```python
from build123d import *

# Parameters (mm, degrees)
BOSS_EXTRUDE1_DEPTH = 10
SKETCH5_W           = 19.453021512
SKETCH5_H           = 38.694970839
BOSS_EXTRUDE2_DEPTH = 85.63051792
SKETCH6_R           = 22
SKETCH6_R_2         = 19.780571117
BOSS_EXTRUDE5_DEPTH = 7.660427645
FILLET10_R          = 2.5
FILLET11_R          = 2.5


with BuildPart() as part:
    # Sketch1 → Boss-Extrude1 (new body)
    with BuildSketch(Plane(origin=(0, 0, 0), x_dir=(1, 0, 0), z_dir=(0, 1, 0))):
        with BuildLine():
            Line((0, 24.518151768), (0, 38.694970839))
            Line((0, 38.694970839), (147.451699193, 38.694970839))
            Line((147.451699193, 38.694970839), (147.451699193, 0))
            Line((147.451699193, 0), (0, 0))
            Line((0, 0), (0, 15.74024552))
            add(Edge.make_bspline(
                [(0, 15.74024552), (2.540846011, 20.138217128), (14.801575787, 5.452312854), (15.995670115, 19.711234682)],
                knots=[0, 0, 0, 0, 1, 1, 1, 1], degree=3))
            add(Edge.make_bspline(
                [(0, 24.518151768), (3.025411482, 20.257839716), (15.777331359, 32.77346932), (15.995670115, 19.711234682)],
                knots=[0, 0, 0, 0, 1, 1, 1, 1], degree=3))
        make_face()
    extrude(amount=BOSS_EXTRUDE1_DEPTH)

    # Sketch5 → Boss-Extrude2 (add)
    with BuildSketch(Plane.XZ):
        with Locations((137.725188437, -19.347485419)):
            Rectangle(SKETCH5_W, SKETCH5_H)
    extrude(amount=BOSS_EXTRUDE2_DEPTH)

    # Sketch6 → Boss-Extrude5 (add)
    with BuildSketch(Plane.ZY.offset(-127.998677681)):
        with Locations(Location((-19.34748542, -65.278, 0), (0, 0, 151.573820003))):
            Circle(SKETCH6_R)
        with Locations(Location((-19.34748542, -65.278, 0), (0, 0, 192.011596254))):
            Circle(SKETCH6_R_2, mode=Mode.SUBTRACT)
    extrude(amount=BOSS_EXTRUDE5_DEPTH)

    # Fillet10
    # the kernel refuses this fillet: 2.5 mm, written as the material it takes off along each edge
    with BuildSketch(Plane(origin=(127.998677681, -65.278, -19.34748542), x_dir=(0, 0.7021921970481064, -0.711987442589231), z_dir=(0, 0.711987442589231, 0.7021921970481064))) as fillet10_piece_1_section:
        with BuildLine():
            CenterArc((19.5, 2.48420608), FILLET10_R, 276.443791757, 83.556208243)
            Line((22, 2.48420608), (22, 0))
            Line((22, 0), (19.780571117, 0))
        make_face()
    fillet10_piece_1 = revolve(axis=Axis((127.998677681, -65.278, -19.34748542), (-1, 0, 0)), revolution_arc=89.20629991, mode=Mode.PRIVATE)
    fillet10_piece_1 = split(fillet10_piece_1, bisect_by=Plane(origin=(127.183421673, -65.278, -38.694970839), z_dir=(0, 0, -1)), keep=Keep.TOP, mode=Mode.PRIVATE)
    add(fillet10_piece_1, mode=Mode.SUBTRACT)

    # Fillet11
    # the kernel refuses this fillet: 2.5 mm, written as the material it takes off along each edge
    with BuildSketch(Plane(origin=(127.998677681, -65.278, -19.34748542), x_dir=(0, -0.7815945319539552, -0.6237868126368795), z_dir=(0, 0.6237868126368795, -0.7815945319539552))) as fillet11_piece_1_section:
        with BuildLine():
            CenterArc((22 - FILLET11_R, FILLET11_R), FILLET11_R, 270, 90)
            Line((22, FILLET11_R), (22, 0))
            Line((22, 0), (22 - FILLET11_R, 0))
        make_face()
    fillet11_piece_1 = revolve(axis=Axis((127.998677681, -65.278, -19.34748542), (-1, 0, 0)), revolution_arc=77.186396047, mode=Mode.PRIVATE)
    fillet11_piece_1 = split(fillet11_piece_1, bisect_by=Plane(origin=(127.364659544, -85.63051792, -19.347486624), z_dir=(0, -1, 0)), keep=Keep.TOP, mode=Mode.PRIVATE)
    add(fillet11_piece_1, mode=Mode.SUBTRACT)


solid = part.part
```
Build history of the part. All positions in model axes, mm. A direction names the side the tool comes from. Give positions to 0.01 mm unless a question says otherwise; leave off trailing zeros. Loops run counter-clockwise (first coordinate to the right, second up) from the corner with the lowest first, then second, coordinate; pieces in that order, holes last. Notation, with made-up numbers: (77.25, 0) -> (127.25, 0) arc R17 ccw to (127.25, 11) -> close; hole circle Ø2 at (-21, 46). An arc over 180 degrees is marked (long way). One line per question, with ' | ' between items.
Q1. Cut at C-C, the plane y = -65. Count the separate pieces of the cut face and the enclosed holes in it, plus the area to 3 significant figures.
Filled sheet:
separate pieces: 3 | enclosed holes: 0 | area: 785 mm²
Q2. Tool access for faces 1 (the flat face through (127.999, -83, -3)), 2 (the flat face through (120.338, -81, -7)), 3 (the flat face through (127.999, -83, -36)): list every direction of +Z, -Z, +X, -X, +Y, -Y with a clear straight run to the whole face (end or side of a thin tool).
Filled sheet:
face 1: +Z, -X, -Y | face 2: +Z, -Z, -X, -Y | face 3: -Z, -X, -Y
Q3. Cut at A-A, the plane y = -77.5. Write the cut outline in (x, z), plus the area to 3 significant figures.
Filled sheet:
outline: (120.34, -37.64) -> (128, -37.64) -> (128, -38.69) -> (147.45, -38.69) -> (147.45, 0) -> (128, 0) -> (128, -1.05) -> (120.34, -1.05) -> (120.34, -3.79) -> (128, -3.79) -> (128, -34.9) -> (120.34, -34.9) -> close | area: 795 mm²
Q4. Pull direction Z, two halves, no side cores. Call faces 4 (the flat face through (127.999, -65, -20)), 5 (the flat face through (129, -23, -38.695)), 6 (the flat face through (127.999, -21, -20)): pulls with the +Z half, pulls with the -Z half, needs draft (parallel to the pull), parting line crosses it, or undercut.
Filled sheet:
face 4: undercut | face 5: pulls with the -Z half | face 6: needs draft
Q5. Cut at D-D, the plane x = 36. Write the cut outline in (y, z).
Filled sheet:
outline: (0, -38.69) -> (10, -38.69) -> (10, 0) -> (0, 0) -> close
Q6. Drill centre lines: line 1 along Y through (x, z) = (123, -18); line 2 along Y through (x, z) = (125, -8.5); line 3 along Y through (x, z) = (131.5, -15). Where is each one in solid material? Low to high. Write a range as [from, to].
Filled sheet:
line 1: y = [-87.24, -85.01], [-45.54, -43.32], [0, 10] | line 2: y = [-84.42, -81.82], [-48.74, -46.14], [0, 10] | line 3: y = [-85.63, 10]
Q7. Drop flat-ended pins along their axis: pin 1 (12 mm diameter, centred on x = 65, z = -32, fed in from -Y); pin 2 (8 mm diameter, centred on y = -81, z = -32.5, fed in from -X); pin 3 (1.3 mm diameter, centred on y = -70, z = 1.5, fed in from +X). Give the stop position or say it passes through.
Filled sheet:
pin 1: stops at y = 0 | pin 2: stops at x = 120.34 | pin 3: stops at x = 128
Q8. Cut at B-B, the plane z = -33. Write the cut outline in (x, y).
Filled sheet:
outline: (0, 0) -> (128, 0) -> (128, -48.03) -> (120.34, -48.03) -> (120.34, -50.96) -> (128, -50.96) -> (128, -79.59) -> (120.34, -79.59) -> (120.34, -82.53) -> (128, -82.53) -> (128, -85.63) -> (147.45, -85.63) -> (147.45, 10) -> (0, 10) -> close
